Autodesk Inventor part; units mm, degrees
ref_plane "YZ Plane" through (0, 0, 0) normal (1, 0, 0) x (0, 1, 0)
ref_plane "XZ Plane" through (0, 0, 0) normal (0, 1, 0) x (-1, 0, 0)
ref_plane "XY Plane" through (0, 0, 0) normal (0, 0, 1) x (1, 0, 0)
sketch "Sketch1" plane through (0, 0, 0) normal (1, 0, 0) x (0, 1, 0)
  circle A0 centre (0, 0) radius 10
  dimension "d0" = 20
extrude "Extrusion1" add sketch "Sketch1" along normal blind 900
sketch "Sketch2" plane through (900, 0, 0) normal (1, 0, 0) x (0, 0, -1)
  circle A0 centre (0, 0) radius 40
  dimension "d3" = 80
extrude "Extrusion2" add sketch "Sketch2" along normal blind 20
fillet "Fillet1" radius 10 1 edges at (900, 0, 40)
fillet "Fillet2" radius 10 1 edges at (900, -10, 0)
properties part number "pneumatic_cylinder_assembly" material "Stainless Steel"
Work out the finished part from the listing and answer in its coordinate system (mm). A direction names the side the tool comes from. Give positions to 0.01 mm unless a question says otherwise; leave off trailing zeros. Loops run counter-clockwise (first coordinate to the right, second up) from the corner with the lowest first, then second, coordinate; pieces in that order, holes last. Notation, with made-up numbers: (-11, 59) - (44, 59) arc R14 ccw to (44, 73) - close; hole circle Ø11 at (31.25, 55). An arc over 180 degrees is marked (long way). Answer in a Markdown table with one row per item.
(1) A tool of negligible diameter and unlimited length cuts with its end or side. For faces 1 (the face through (900, -20, -6)), 2 (the face through (920, 1, 1)), from which of +Z, -Z, +X, -X, +Y, -Y can it reach the whole face along a straight path? Write none if from no direction.
Results list:
| item | result |
|---|---|
| face 1 | -X |
| face 2 | +Z, -Z, +X, +Y, -Y |
(2) Consider L1, parallel to X at y = 19.5, z = 6; L2, parallel to Z at x = 76, y = -5; L3, parallel to Y at x = 519, z = -4.5. Determine where each line is inside the solid, lowest interval first. Write a range as [from, to].
Results list:
| item | result |
|---|---|
| L1 | x = [900, 920] |
| L2 | z = [-8.66, 8.66] |
| L3 | y = [-8.93, 8.93] |
(3) Section A-A (z = 0) is taken. Give the vertices of the cut face in (x, y), and give its area (3 significant figures).
Results list:
| item | result |
|---|---|
| outline | (0, -10) - (890, -10) arc R10 cw to (900, -20) - (900, -30) arc R10 ccw to (910, -40) - (920, -40) - (920, 40) - (910, 40) arc R10 ccw to (900, 30) - (900, 20) arc R10 cw to (890, 10) - (0, 10) - close |
| area | 19,600 mm² |
(4) Section C-C (x = 75) is taken. Give the vertices of the cut face in (y, z).
Results list:
| item | result |
|---|---|
| outline | circle Ø20 at (0, 0) |
(5) Flat-ended cylindrical pins translate along their axes: pin 1 Ø1 at (x, z) = (292, 6) entering from -Y; pin 2 Ø2 at (y, z) = (19, -19.5) entering from -X; pin 3 Ø6 at (x, y) = (577, 14.5) entering from -Z (1 decimal); pin 4 Ø1.5 at (x, y) = (713.5, 9) entering from +Z. Find the tip coordinate at first contact, or state that the pin passes through.
Results list:
| item | result |
|---|---|
| pin 1 | stops at y = -8.35 |
| pin 2 | stops at x = 900 |
| pin 3 | passes through |
| pin 4 | stops at z = 5.65 |
